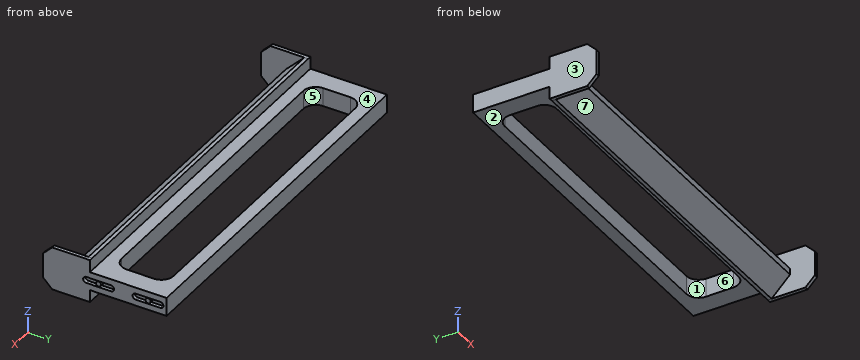
```python
from build123d import *

# Parameters (mm, degrees)
F1_DEPTH       = 17.5
F1_DEPTH_BACK  = 17.5
F2_SIZE        = 15
F3_SIZE        = 7.5
F5_W           = 3
F5_H           = 92.5
F6_DEPTH       = 0.01
F7_W           = 3
F7_H           = 92.5
F8_DEPTH       = 0.01
F4_R           = 2.1
F9_DEPTH       = 3
F11_DEPTH      = 10
F13_DEPTH      = 10
F15_DEPTH      = 25
F16_W          = 295
F16_H          = 62
F17_DEPTH      = 10
F17_DEPTH_BACK = 25
F18_W          = 295
F18_H          = 62
F19_DEPTH      = 10
F19_DEPTH_BACK = 25


with BuildPart() as f1:
    # F0 (on Top) → F1 (new body, two sides)
    with BuildSketch(Plane.XY) as f1_sk:
        Polygon((147.5, -50), (147.5, 50), (-147.5, 50), (-147.5, -50), (-144.5, -50), (-144.5, -30), (144.5, -30), (144.5, -50), align=None)
    extrude(amount=F1_DEPTH)
    extrude(f1_sk.sketch, amount=-F1_DEPTH_BACK)

    # F2
    f2_edges = [f1.edges().sort_by_distance(p)[0] for p in [
        (0, -30, 17.5),
        (0, -30, -17.5),
    ]]
    chamfer(f2_edges, length=F2_SIZE)

    # F3
    f3_edges = [f1.edges().sort_by_distance(p)[0] for p in [
        (146, -50, 17.5),
        (146, -50, -17.5),
        (-146, -50, 17.5),
        (-146, -50, -17.5),
    ]]
    chamfer(f3_edges, length=F3_SIZE)

    # F5 (on face) → F6 (join)
    with BuildSketch(Plane.XY.offset(17.5)):
        with Locations((-146, 3.75)):
            Rectangle(F5_W, F5_H)
        with Locations((146, 3.75)):
            Rectangle(F5_W, F5_H)
    extrude(amount=F6_DEPTH)

    # F7 (on face) → F8 (join)
    with BuildSketch(Plane(origin=(0, 0, -17.5), x_dir=(1, 0, 0), z_dir=(0, 0, -1))):
        with Locations((-146, -3.75)):
            Rectangle(F7_W, F7_H)
        with Locations((146, -3.75)):
            Rectangle(F7_W, F7_H)
    extrude(amount=F8_DEPTH)

    # F4 (on face) → F9 (cut)
    with BuildSketch(Plane.YZ.offset(147.5)):
        with BuildLine():
            ThreePointArc((47.5, 0), (46.767766953, 1.767766953), (45, 2.5))
            Line((45, 2.5), (25, 2.5))
            ThreePointArc((25, 2.5), (23.232233047, 1.767766953), (22.5, 0))
            ThreePointArc((22.5, 0), (23.232233047, -1.767766953), (25, -2.5))
            Line((25, -2.5), (45, -2.5))
            ThreePointArc((45, -2.5), (46.767766953, -1.767766953), (47.5, 0))
        make_face()
        with Locations((35, 0)):
            Circle(F4_R, mode=Mode.SUBTRACT)
        with BuildLine():
            ThreePointArc((7.5, 0), (6.767766953, 1.767766953), (5, 2.5))
            Line((5, 2.5), (-15, 2.5))
            ThreePointArc((-15, 2.5), (-16.767766953, 1.767766953), (-17.5, 0))
            ThreePointArc((-17.5, 0), (-16.767766953, -1.767766953), (-15, -2.5))
            Line((-15, -2.5), (5, -2.5))
            ThreePointArc((5, -2.5), (6.767766953, -1.767766953), (7.5, 0))
        make_face()
        with Locations((-5, 0)):
            Circle(F4_R, mode=Mode.SUBTRACT)
    extrude(amount=-F9_DEPTH, mode=Mode.SUBTRACT)

    # F10 (on face) → F11 (cut)
    with BuildSketch(Plane.XY.offset(17.5)):
        with BuildLine():
            Line((141.5, 50), (-141.5, 50))
            Line((-141.5, 50), (-141.5, -2))
            ThreePointArc((-141.5, -2), (-138.5710678119, -9.0710678119), (-131.5, -12))
            Line((-131.5, -12), (131.5, -12))
            ThreePointArc((131.5, -12), (138.5710678119, -9.0710678119), (141.5, -2))
            Line((141.5, -2), (141.5, 50))
        make_face()
    extrude(amount=-F11_DEPTH, mode=Mode.SUBTRACT)

    # F12 (on face) → F13 (cut)
    with BuildSketch(Plane(origin=(0, 0, -17.5), x_dir=(1, 0, 0), z_dir=(0, 0, -1))):
        with BuildLine():
            Line((141.5, -50), (141.5, 2))
            ThreePointArc((141.5, 2), (138.5710678119, 9.0710678119), (131.5, 12))
            Line((131.5, 12), (-131.5, 12))
            ThreePointArc((-131.5, 12), (-138.5710678119, 9.0710678119), (-141.5, 2))
            Line((-141.5, 2), (-141.5, -50))
            Line((-141.5, -50), (141.5, -50))
        make_face()
    extrude(amount=-F13_DEPTH, mode=Mode.SUBTRACT)

    # F14 (on face) → F15 (cut)
    with BuildSketch(Plane.XY.offset(7.5)):
        with BuildLine():
            Line((121.5, 40), (-121.5, 40))
            ThreePointArc((-121.5, 40), (-128.5710678119, 37.0710678119), (-131.5, 30))
            Line((-131.5, 30), (-131.5, 8))
            ThreePointArc((-131.5, 8), (-128.5710678119, 0.9289321881), (-121.5, -2))
            Line((-121.5, -2), (121.5, -2))
            ThreePointArc((121.5, -2), (128.5710678119, 0.9289321881), (131.5, 8))
            Line((131.5, 8), (131.5, 30))
            ThreePointArc((131.5, 30), (128.5710678119, 37.0710678119), (121.5, 40))
        make_face()
    extrude(amount=-F15_DEPTH, mode=Mode.SUBTRACT)

    # F16 (on face) → F17 (cut, two sides)
    with BuildSketch(Plane.XY.offset(17.5)) as f17_sk:
        with Locations((0, 19)):
            Rectangle(F16_W, F16_H)
    extrude(amount=-F17_DEPTH, mode=Mode.SUBTRACT)
    extrude(f17_sk.sketch, amount=F17_DEPTH_BACK, mode=Mode.SUBTRACT)

    # F18 (on face) → F19 (cut, two sides)
    with BuildSketch(Plane(origin=(0, 0, -17.5), x_dir=(1, 0, 0), z_dir=(0, 0, -1))) as f19_sk:
        with Locations((0, -19)):
            Rectangle(F18_W, F18_H)
    extrude(amount=-F19_DEPTH, mode=Mode.SUBTRACT)
    extrude(f19_sk.sketch, amount=F19_DEPTH_BACK, mode=Mode.SUBTRACT)


solid = f1.part
```
Model file for the job. Use its own axes, mm. Face numbers are marked on the shaded views. A direction names the side the tool comes from. Give positions to 0.01 mm unless a question says otherwise; leave off trailing zeros. Write each loop counter-clockwise with the first axis right and the second up, starting at its lowest first coordinate (ties: lowest second). Pieces come first, ordered by that corner, then holes. Notation, with made-up numbers: M 13.25,68.25 L 63.25,68.25 A26 ccw 63.25,106.25 Z; hole C 5.25,73.25 d5. An arc over 180 degrees is marked long. Use a Markdown table: item, result.
1) Pull direction Y, two halves, no side cores. Call the marked faces 4, 5, 6 and 7: +Y half, -Y half, draft (parallel to the pull), parting line (faces both ways), or undercut.
Responses:
| item | result |
|---|---|
| face 4 | draft |
| face 5 | undercut |
| face 6 | undercut |
| face 7 | -Y half |
2) Drill centre lines: line 1 (X direction, y = 18, z = -2); line 2 (Y direction, x = 67.5, z = -2); line 3 (X direction, y = -26, z = -14). Where is each one in solid material? Low to high. Write a range as from..to.
Responses:
| item | result |
|---|---|
| line 1 | x = -147.5..-131.5, 131.5..147.5 |
| line 2 | y = -30..-2, 40..50 |
| line 3 | x = -147.5..-144.5, 144.5..147.5 |
3) Cut at A-A (x = 33). List the corners of the cut face in (y, z), and give its area (3 significant figures).
Responses:
| item | result |
|---|---|
| outline | M -30,-2.5 L -15,-17.5 L -12,-17.5 L -12,-7.5 L -2,-7.5 L -2,7.5 L -12,7.5 L -12,17.5 L -15,17.5 L -30,2.5 Z; M 40,-7.5 L 50,-7.5 L 50,7.5 L 40,7.5 Z |
| area | 705 mm2 |
4) Pin check, flat tips, straight feed: pin 1 (3.5 mm diameter, centred on x = 145.5, y = -1, fed in from -Z); pin 2 (8 mm diameter, centred on x = -8.5, y = -1, fed in from +Z); pin 3 (2.5 mm diameter, centred on x = 20, y = -13, fed in from -Z). Stop position of each tip, or through.
Responses:
| item | result |
|---|---|
| pin 1 | stops at z = -7.5 |
| pin 2 | stops at z = 7.5 |
| pin 3 | stops at z = -17.5 |
5) Tool access for the marked faces 1, 2 and 3: list every direction of +Z, -Z, +X, -X, +Y, -Y with a clear straight run to the whole face (end or side of a thin tool).
Responses:
| item | result |
|---|---|
| face 1 | +Z, -Z |
| face 2 | -Z, +X, -X, +Y |
| face 3 | +Z, -Z, -X, +Y, -Y |
6) Cut at B-B (y = -26). List the corners of the cut face in (x, z), and give its area (3 significant figures).
Responses:
| item | result |
|---|---|
| outline | M -147.5,-17.51 L -144.5,-17.51 L -144.5,-6.5 L 144.5,-6.5 L 144.5,-17.51 L 147.5,-17.51 L 147.5,17.51 L 144.5,17.51 L 144.5,6.5 L -144.5,6.5 L -144.5,17.51 L -147.5,17.51 Z |
| area | 3,970 mm2 |
